For this review, take the finished solid that the model builds, in its own axes (mm). A direction names the side the tool comes from. Coordinates: 2 decimals unless noted, no trailing zeros. Write each loop counter-clockwise with the first axis right and the second up, starting at its lowest first coordinate (ties: lowest second). Pieces come first, ordered by that corner, then holes. Notation, with made-up numbers: M -3,64.25 L 19,64.25 A4 cw 19,70.25 Z; hole C 68,51 d5. An arc over 180 degrees is marked long. One line per question, with ' | ' between items.
from build123d import *

# Parameters (mm, degrees)
PAD_DEPTH     = 2
SKETCH002_W   = 20
SKETCH002_H   = 20
PAD001_DEPTH  = 50
SKETCH004_R   = 8
POCKET_DEPTH  = 52.001
PAD002_DEPTH  = 0.5
SKETCH010_R   = 3.8
SKETCH010_R_2 = 1.4
PAD003_DEPTH  = 5
SKETCH011_R   = 3
SKETCH011_R_2 = 1.4
PAD004_DEPTH  = 20
SKETCH012_W   = 5
SKETCH012_H   = 20
SKETCH012_R   = 0.9
SKETCH012_W_2 = 10
SKETCH012_H_2 = 5
PAD005_DEPTH  = 10
SKETCH013_R   = 3
SKETCH013_R_2 = 1.4
PAD006_DEPTH  = 3


with BuildPart() as part:
    # Sketch → Pad (new body)
    with BuildSketch(Plane.XY):
        with BuildLine():
            Line((-65, 70), (65, 70))
            ThreePointArc((70, 65), (68.535534, 68.535534), (65, 70))
            Line((70, 65), (70, -65))
            ThreePointArc((65, -70), (68.535534, -68.535534), (70, -65))
            Line((65, -70), (-65, -70))
            ThreePointArc((-70, -65), (-68.535534, -68.535534), (-65, -70))
            Line((-70, -65), (-70, 65))
            ThreePointArc((-65, 70), (-68.535534, 68.535534), (-70, 65))
        make_face()
    extrude(amount=PAD_DEPTH)

    # Sketch002 → Pad001 (new body)
    with BuildSketch(Plane.XY.offset(2)):
        with Locations((-40, 30)):
            Rectangle(SKETCH002_W, SKETCH002_H)
        with Locations((4, -55)):
            Rectangle(SKETCH002_W, SKETCH002_H)
        with Locations((40, 30)):
            Rectangle(SKETCH002_W, SKETCH002_H)
    extrude(amount=PAD001_DEPTH)

    # Sketch004 → Pocket (cut, through all)
    with BuildSketch(Plane.XY.offset(52)):
        with Locations((-40, 30)):
            Circle(SKETCH004_R)
        with Locations((40, 30)):
            Circle(SKETCH004_R)
        with Locations((4, -55)):
            Circle(SKETCH004_R)
    extrude(amount=-POCKET_DEPTH, mode=Mode.SUBTRACT)

    # Sketch001 → Pad002 (new body)
    with BuildSketch(Plane.XY.offset(2)):
        with BuildLine():
            Line((2.307479, 19.099802), (62.307479, 19.099802))
            ThreePointArc((64.307479, 17.099802), (63.721693, 18.514015), (62.307479, 19.099802))
            Line((64.307479, 17.099802), (64.307479, -22.900198))
            ThreePointArc((62.307479, -24.900198), (63.721693, -24.314412), (64.307479, -22.900198))
            Line((62.307479, -24.900198), (2.307479, -24.900198))
            ThreePointArc((0.307479, -22.900198), (0.893266, -24.314412), (2.307479, -24.900198))
            Line((0.307479, -22.900198), (0.307479, 17.099802))
            ThreePointArc((2.307479, 19.099802), (0.893266, 18.514015), (0.307479, 17.099802))
        make_face()
        with BuildLine():
            Line((3.307479, 18.099802), (61.307479, 18.099802))
            ThreePointArc((63.307479, 16.099802), (62.721693, 17.514015), (61.307479, 18.099802))
            Line((63.307479, 16.099802), (63.307479, -21.900198))
            ThreePointArc((61.307479, -23.900198), (62.721693, -23.314412), (63.307479, -21.900198))
            Line((61.307479, -23.900198), (3.307479, -23.900198))
            ThreePointArc((1.307479, -21.900198), (1.893266, -23.314412), (3.307479, -23.900198))
            Line((1.307479, -21.900198), (1.307479, 16.099802))
            ThreePointArc((3.307479, 18.099802), (1.893266, 17.514015), (1.307479, 16.099802))
        make_face(mode=Mode.SUBTRACT)
        with BuildLine():
            Line((16.890482, -26.060452), (62.890482, -26.060452))
            ThreePointArc((64.890482, -28.060452), (64.304696, -26.646238), (62.890482, -26.060452))
            Line((64.890482, -28.060452), (64.890482, -64.060452))
            ThreePointArc((62.890482, -66.060452), (64.304696, -65.474665), (64.890482, -64.060452))
            Line((62.890482, -66.060452), (16.890482, -66.060452))
            ThreePointArc((14.890482, -64.060452), (15.476269, -65.474665), (16.890482, -66.060452))
            Line((14.890482, -64.060452), (14.890482, -28.060452))
            ThreePointArc((16.890482, -26.060452), (15.476269, -26.646238), (14.890482, -28.060452))
        make_face()
        with BuildLine():
            Line((17.890482, -27.060452), (61.890482, -27.060452))
            ThreePointArc((63.890482, -29.060452), (63.304696, -27.646238), (61.890482, -27.060452))
            Line((63.890482, -29.060452), (63.890482, -63.060452))
            ThreePointArc((61.890482, -65.060452), (63.304696, -64.474665), (63.890482, -63.060452))
            Line((61.890482, -65.060452), (17.890482, -65.060452))
            ThreePointArc((15.890482, -63.060452), (16.476269, -64.474665), (17.890482, -65.060452))
            Line((15.890482, -63.060452), (15.890482, -29.060452))
            ThreePointArc((17.890482, -27.060452), (16.476269, -27.646238), (15.890482, -29.060452))
        make_face(mode=Mode.SUBTRACT)
        with BuildLine():
            Line((-64.647393, 18.925724), (-11.647393, 18.925724))
            ThreePointArc((-9.647393, 16.925724), (-10.233179, 18.339937), (-11.647393, 18.925724))
            Line((-9.647393, -22.074276), (-9.647393, 16.925724))
            Line((-3.647393, -22.074276), (-9.647393, -22.074276))
            Line((-3.647393, -29.074276), (-3.647393, -22.074276))
            Line((-9.647393, -29.074276), (-3.647393, -29.074276))
            Line((-9.647393, -64.074276), (-9.647393, -29.074276))
            ThreePointArc((-11.647393, -66.074276), (-10.233179, -65.48849), (-9.647393, -64.074276))
            Line((-11.647393, -66.074276), (-64.647393, -66.074276))
            ThreePointArc((-66.647393, -64.074276), (-66.061606, -65.48849), (-64.647393, -66.074276))
            Line((-66.647393, -64.074276), (-66.647393, 16.925724))
            ThreePointArc((-64.647393, 18.925724), (-66.061606, 18.339937), (-66.647393, 16.925724))
        make_face()
        with BuildLine():
            Line((-63.647393, 17.925724), (-12.647393, 17.925724))
            ThreePointArc((-10.647393, 15.925724), (-11.233179, 17.339937), (-12.647393, 17.925724))
            Line((-10.647393, 15.925724), (-10.647393, -63.074276))
            ThreePointArc((-12.647393, -65.074276), (-11.233179, -64.48849), (-10.647393, -63.074276))
            Line((-12.647393, -65.074276), (-63.647393, -65.074276))
            ThreePointArc((-65.647393, -63.074276), (-65.061606, -64.48849), (-63.647393, -65.074276))
            Line((-65.647393, -63.074276), (-65.647393, 15.925724))
            ThreePointArc((-63.647393, 17.925724), (-65.061606, 17.339937), (-65.647393, 15.925724))
        make_face(mode=Mode.SUBTRACT)
        with BuildLine():
            Line((2.324005, 63.83459), (62.324005, 63.83459))
            ThreePointArc((64.324005, 61.83459), (63.738218, 63.248804), (62.324005, 63.83459))
            Line((64.324005, 61.83459), (64.324005, 43.83459))
            ThreePointArc((62.324005, 41.83459), (63.738218, 42.420377), (64.324005, 43.83459))
            Line((62.324005, 41.83459), (2.324005, 41.83459))
            ThreePointArc((0.324005, 43.83459), (0.909791, 42.420377), (2.324005, 41.83459))
            Line((0.324005, 43.83459), (0.324005, 61.83459))
            ThreePointArc((2.324005, 63.83459), (0.909791, 63.248804), (0.324005, 61.83459))
        make_face()
        with BuildLine():
            Line((3.324005, 62.83459), (61.324005, 62.83459))
            ThreePointArc((63.324005, 60.83459), (62.738218, 62.248804), (61.324005, 62.83459))
            Line((63.324005, 60.83459), (63.324005, 44.83459))
            ThreePointArc((61.324005, 42.83459), (62.738218, 43.420377), (63.324005, 44.83459))
            Line((61.324005, 42.83459), (3.324005, 42.83459))
            ThreePointArc((1.324005, 44.83459), (1.909791, 43.420377), (3.324005, 42.83459))
            Line((1.324005, 44.83459), (1.324005, 60.83459))
            ThreePointArc((3.324005, 62.83459), (1.909791, 62.248804), (1.324005, 60.83459))
        make_face(mode=Mode.SUBTRACT)
    extrude(amount=PAD002_DEPTH)

    # Sketch010 → Pad003 (new body)
    with BuildSketch(Plane.XY.offset(2)):
        with Locations((-22.147393, -61.074276)):
            Circle(SKETCH010_R)
        with Locations((-22.147393, -61.074276)):
            Circle(SKETCH010_R_2, mode=Mode.SUBTRACT)
        with Locations((-47.147393, -7.074276)):
            Circle(SKETCH010_R)
        with Locations((-47.147393, -7.074276)):
            Circle(SKETCH010_R_2, mode=Mode.SUBTRACT)
    extrude(amount=PAD003_DEPTH)

    # Sketch011 → Pad004 (new body)
    with BuildSketch(Plane.XY.offset(2)):
        with Locations((17.810321, -30.060452)):
            Circle(SKETCH011_R)
        with Locations((17.810321, -30.060452)):
            Circle(SKETCH011_R_2, mode=Mode.SUBTRACT)
        with Locations((61.810321, -30.060452)):
            Circle(SKETCH011_R)
        with Locations((61.810321, -30.060452)):
            Circle(SKETCH011_R_2, mode=Mode.SUBTRACT)
        with Locations((61.810321, -62.060452)):
            Circle(SKETCH011_R)
        with Locations((61.810321, -62.060452)):
            Circle(SKETCH011_R_2, mode=Mode.SUBTRACT)
        with Locations((17.810321, -62.060452)):
            Circle(SKETCH011_R)
        with Locations((17.810321, -62.060452)):
            Circle(SKETCH011_R_2, mode=Mode.SUBTRACT)
    extrude(amount=PAD004_DEPTH)

    # Sketch012 → Pad005 (new body)
    with BuildSketch(Plane.XY.offset(2)):
        with Locations((23.828853, 52.895568)):
            Rectangle(SKETCH012_W, SKETCH012_H)
        with Locations((23.828853, 61.145568)):
            Circle(SKETCH012_R, mode=Mode.SUBTRACT)
        with Locations((23.828853, 44.645568)):
            Circle(SKETCH012_R, mode=Mode.SUBTRACT)
        with Locations((58.328853, 60.395568)):
            Rectangle(SKETCH012_W_2, SKETCH012_H_2)
        with Locations((61.328853, 61.145568)):
            Circle(SKETCH012_R, mode=Mode.SUBTRACT)
        with Locations((58.328853, 45.395568)):
            Rectangle(SKETCH012_W_2, SKETCH012_H_2)
        with Locations((61.328853, 44.645568)):
            Circle(SKETCH012_R, mode=Mode.SUBTRACT)
    extrude(amount=PAD005_DEPTH)

    # Sketch013 → Pad006 (new body)
    with BuildSketch(Plane.XY.offset(2)):
        with Locations((20.307479, 14.099802)):
            Circle(SKETCH013_R)
        with Locations((20.307479, 14.099802)):
            Circle(SKETCH013_R_2, mode=Mode.SUBTRACT)
        with Locations((20.307479, -19.900198)):
            Circle(SKETCH013_R)
        with Locations((20.307479, -19.900198)):
            Circle(SKETCH013_R_2, mode=Mode.SUBTRACT)
        with Locations((57.307479, 9.599802)):
            Circle(SKETCH013_R)
        with Locations((57.307479, 9.599802)):
            Circle(SKETCH013_R_2, mode=Mode.SUBTRACT)
        with Locations((57.307479, -15.400198)):
            Circle(SKETCH013_R)
        with Locations((57.307479, -15.400198)):
            Circle(SKETCH013_R_2, mode=Mode.SUBTRACT)
    extrude(amount=PAD006_DEPTH)


solid = part.part
1) We need section B-B on y = -55. State the section outline as (x, z) points, then the cut area to 3 significant figures.
Responses:
outline: M -70,0 L -4,0 L -4,52 L -6,52 L -6,2 L -9.65,2 L -9.65,2.5 L -10.65,2.5 L -10.65,2 L -65.65,2 L -65.65,2.5 L -66.65,2.5 L -66.65,2 L -70,2 Z; M 12,0 L 70,0 L 70,2 L 64.89,2 L 64.89,2.5 L 63.89,2.5 L 63.89,2 L 15.89,2 L 15.89,2.5 L 14.89,2.5 L 14.89,2 L 14,2 L 14,52 L 12,52 Z | area: 450 mm^2
2) The part is to be moulded in two halves that separate along X. For faces 5 (the flat face through (63.329, 60, 7)), 6 (the flat face through (-47, -9, 7)), 7 (the cylindrical face through (55.1, -13.37, 3.48)), say which applies: +X half, -X half, draft (parallel to the pull), parting line (faces both ways), or undercut.
Responses:
face 5: +X half | face 6: draft | face 7: undercut
3) Machinability: for faces 1 (the cylindrical face through (21.92, -17.37, 3.48)), 2 (the flat face through (-30, 30, 27)), 3 (the flat face through (22, 13, 5)), 4 (the flat face through (58, 62.896, 7)), which of the approach directions +Z, -Z, +X, -X, +Y, -Y give a long, thin tool a straight path to every point of the face, cutting with its end or side? Answer none if there is none.
Responses:
face 1: +Z | face 2: +Z, +Y, -Y | face 3: +Z, +X, -X | face 4: +Z, +X, -X, +Y
4) We need section D-D on y = 25.5. State the section outline as (x, z) points, then the cut area to 3 significant figures.
Responses:
outline: M -70,0 L -46.61,0 L -46.61,52 L -50,52 L -50,2 L -70,2 Z; M -33.39,0 L 33.39,0 L 33.39,52 L 30,52 L 30,2 L -30,2 L -30,52 L -33.39,52 Z; M 46.61,0 L 70,0 L 70,2 L 50,2 L 50,52 L 46.61,52 Z | area: 904 mm^2
5) We need section C-C on z = 16. State how many separate pieces and enclosed holes the cut face has, then the cut area to 3 significant figures.
Responses:
separate pieces: 7 | enclosed holes: 7 | area: 685 mm^2
6) We need section A-A on x = -40. State the section outline as (y, z) points, then the cut area to 3 significant figures.
Responses:
outline: M -70,0 L 22,0 L 22,52 L 20,52 L 20,2 L 18.93,2 L 18.93,2.5 L 17.93,2.5 L 17.93,2 L -65.07,2 L -65.07,2.5 L -66.07,2.5 L -66.07,2 L -70,2 Z; M 38,0 L 70,0 L 70,2 L 40,2 L 40,52 L 38,52 Z | area: 449 mm^2
7) Insertion check: pin 1 Ø8 at (x, z) = (22, 13.5) entering from -Y; pin 2 Ø0.6 at (x, z) = (44.5, 2.5) entering from +Y; pin 3 Ø6 at (y, z) = (29, 30.5) entering from -X. Each pin has a flat end and moves straight along its axis. Give the tip position at first contact, or say it passes through.
Responses:
pin 1: y = -65.05 | pin 2: y = 63.83 | pin 3: x = -50
8) To check wall thickness, follow line 1 along Y through (x, z) = (55, 8.5); line 2 along X through (y, z) = (29.5, 41); line 3 along X through (y, z) = (47.5, 6.5). State the ranges of each line that lie inside material, in increasing order. Write a range as [from, to].
Responses:
line 1: [42.9, 47.9], [57.9, 62.9] | line 2: [-50, -47.98], [-32.02, -30], [30, 32.02], [47.98, 50] | line 3: [21.33, 26.33], [53.33, 63.33]
